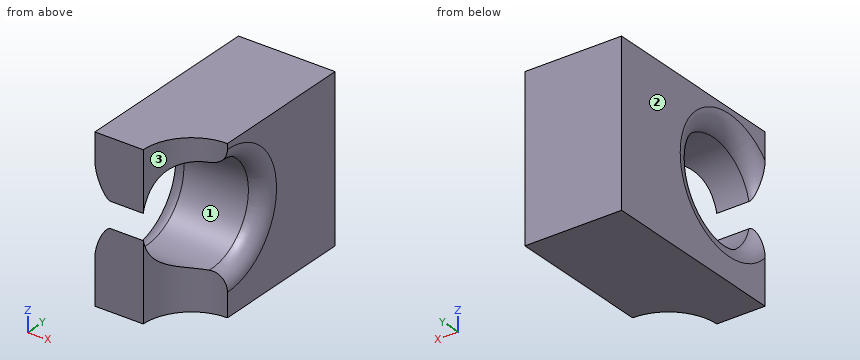
```python
from build123d import *

# Parameters (mm, degrees)
F1_DEPTH = 50
F2_R     = 15.5
F3_DEPTH = 70
F4_R     = 5


with BuildPart() as f1:
    # F0 (on Top) → F1 (new body)
    with BuildSketch(Plane.XY):
        with BuildLine():
            Line((-25.2489881364, 31.0668002069), (-25.2489881364, -28.9331997931))
            Line((-25.2489881364, -28.9331997931), (-10.2489881364, -28.9331997931))
            ThreePointArc((-10.2489881364, -28.9331997931), (-5.8555898542, -18.3265980753), (4.7510118636, -13.9331997931))
            Line((4.7510118636, -13.9331997931), (4.7510118636, 31.0668002069))
            Line((4.7510118636, 31.0668002069), (-25.2489881364, 31.0668002069))
        make_face()
    extrude(amount=F1_DEPTH)

    # F2 (on face) → F3 (cut)
    with BuildSketch(Plane.YZ.offset(4.7510118636)):
        with Locations((-13.9331997931, 27.8249997646)):
            Circle(F2_R)
    extrude(amount=-F3_DEPTH, mode=Mode.SUBTRACT)

    # F4
    f4_edges = [f1.edges().sort_by_distance(p)[0] for p in [
        (4.751012, 1.5668, 27.825),
        (-25.248988, 1.5668, 27.825),
    ]]
    fillet(f4_edges, radius=F4_R)


solid = f1.part
```
CAD build for the part. Positions are in the model's coordinates, mm. Face numbers are marked on the shaded views. Round coordinates to 2 decimals unless told otherwise and drop trailing zeros. Order: outer loops, then holes, each group sorted by start corner. A loop starts at its lowest first (then second) coordinate and runs counter-clockwise, first axis right, second up. Notation, with made-up numbers: (13.5, -22.5) - (67.5, -22.5) arc R19 cw to (67.5, 14.5) - close; hole circle Ø8 at (83.25, 35.5). An arc over 180 degrees is marked (long way). Use CSV: the item, a comma, the result in double quotes. Start each with the question number.
1) Two-plate mould, pull along Y, no slides. Class the marked faces 1, 2 and 3: pulls with the +Y half, pulls with the -Y half, needs draft (parallel to the pull), parting line crosses it, or undercut.
2) Saw through at C-C (x = 2.5). List the corners of the cut face in (y, z) (3 decimals).
3) Saw through at A-A (x = -17). List the corners of the cut face in (y, z) (3 decimals), and give its area (3 significant figures).
4) Saw through at B-B (z = 4). List the corners of the cut face in (x, y), and give its area (3 significant figures).
5) Pin check, flat tip, straight feed: pin 1 Ø1 at (x, y) = (-3, 3.5) entering from -Z. Stop position of the tip, or through.
6) Wall check: L1, parallel to Y at x = -23, z = 37; L2, parallel to Z at x = -9.5, y = -16.5; L3, parallel to Z at x = -20, y = -11. Give the ranges that are in metal, low to high. Write a range as [from, to].
Values follow:
1,face 1,"undercut"
1,face 2,"needs draft"
1,face 3,"pulls with the -Y half"
2,outline,"(-14.103, 0) - (31.067, 0) - (31.067, 50) - (-14.103, 50) - (-14.103, 44.148) arc R16.324 cw (long way) to (-14.103, 11.502) - close"
3,outline,"(-28.933, 0) - (31.067, 0) - (31.067, 50) - (-28.933, 50) - (-28.933, 31.73) arc R15.5 cw (long way) to (-28.933, 23.92) - close"
3,area,"2,250 mm2"
4,outline,"(-25.25, -28.93) - (-10.25, -28.93) arc R15 cw to (4.75, -13.93) - (4.75, 31.07) - (-25.25, 31.07) - close"
4,area,"1,620 mm2"
5,pin 1,"stops at z = 0"
6,L1,"y = [-28.93, -27.44], [-0.43, 31.07]"
6,L2,"z = [0, 12.54], [43.11, 50]"
6,L3,"z = [0, 12.61], [43.04, 50]"
